from build123d import *

# Parameters (mm, degrees)
SKETCH_W        = 40
SKETCH_H        = 50
PAD_DEPTH       = 7
SKETCH001_R     = 2.5
SKETCH001_R_2   = 5
POCKET_DEPTH    = 7.001
POCKET001_DEPTH = 5
SKETCH003_W     = 11.6
SKETCH003_H     = 1
PAD001_DEPTH    = 50
SKETCH004_R     = 3
POCKET002_DEPTH = 8.001
SKETCH005_R     = 6
POCKET003_DEPTH = 1
CHAMFER_SIZE    = 2.49
FILLET_R        = 4
POCKET004_DEPTH = 8.001
FILLET001_R     = 1


with BuildPart() as part:
    # Sketch → Pad (new body)
    with BuildSketch(Plane.XY):
        with Locations((10, 0)):
            Rectangle(SKETCH_W, SKETCH_H)
    extrude(amount=PAD_DEPTH)

    # Sketch001 (on Face6 of Pad) → Pocket (cut, through all)
    with BuildSketch(Plane.XY.offset(7)):
        with Locations((21.50647, 18.25)):
            Circle(SKETCH001_R)
        with Locations((21.50647, -18.25)):
            Circle(SKETCH001_R)
        with Locations((22, 0)):
            Circle(SKETCH001_R_2)
    extrude(amount=-POCKET_DEPTH, mode=Mode.SUBTRACT)

    # Sketch002 (on Face4 of Pocket) → Pocket001 (cut)
    with BuildSketch(Plane(origin=(0, 0, 0), x_dir=(1, 0, 0), z_dir=(0, 0, -1))):
        Polygon((19.052731, 14), (23.960208, 14), (26.413947, 18.25), (23.960208, 22.5), (19.052731, 22.5), (16.598992, 18.25), align=None)
        Polygon((19.052731, -22.5), (23.960208, -22.5), (26.413947, -18.25), (23.960208, -14), (19.052731, -14), (16.598992, -18.25), align=None)
    extrude(amount=-POCKET001_DEPTH, mode=Mode.SUBTRACT)

    # Sketch003 (on Face1 of Pocket001) → Pad001 (join)
    with BuildSketch(Plane(origin=(0, 25, 0), x_dir=(-1, 0, 0), z_dir=(0, 1, 0))):
        with Locations((0, -0.5)):
            Rectangle(SKETCH003_W, SKETCH003_H)
    extrude(amount=-PAD001_DEPTH)

    # Sketch004 (on Face5 of Pad001) → Pocket002 (cut, through all)
    with BuildSketch(Plane.XY.offset(7)):
        with Locations((0, 15)):
            Circle(SKETCH004_R)
        with Locations((0, -15)):
            Circle(SKETCH004_R)
    extrude(amount=-POCKET002_DEPTH, mode=Mode.SUBTRACT)

    # Sketch005 (on Face5 of Pocket002) → Pocket003 (cut)
    with BuildSketch(Plane.XY.offset(7)):
        with Locations((0, 15)):
            Circle(SKETCH005_R)
        with Locations((0, -15)):
            Circle(SKETCH005_R)
    extrude(amount=-POCKET003_DEPTH, mode=Mode.SUBTRACT)

    # Chamfer
    chamfer_edges = [part.edges().sort_by_distance(p)[0] for p in [
        (-3, -15, 6),
        (-3, 15, 6),
    ]]
    chamfer(chamfer_edges, length=CHAMFER_SIZE)

    # Fillet
    fillet_edges = [part.edges().sort_by_distance(p)[0] for p in [
        (-10, -25, 3.5),
        (30, -25, 3.5),
        (30, 25, 3.5),
        (-10, 25, 3.5),
    ]]
    fillet(fillet_edges, radius=FILLET_R)

    # Sketch006 (on Face1 of Fillet) → Pocket004 (cut, through all)
    with BuildSketch(Plane.XY.offset(7)):
        with BuildLine():
            ThreePointArc((-10, 15), (-6.785937, 6.309375), (0, 0))
            ThreePointArc((0, 0), (-6.785937, -6.309375), (-10, -15))
            Line((-10, 15), (-10, -15))
        make_face()
    extrude(amount=-POCKET004_DEPTH, mode=Mode.SUBTRACT)

    # Fillet001
    fillet001_edges = [part.edges().sort_by_distance(p)[0] for p in [
        (30, 0, 7),
    ]]
    fillet(fillet001_edges, radius=FILLET001_R)


solid = part.part
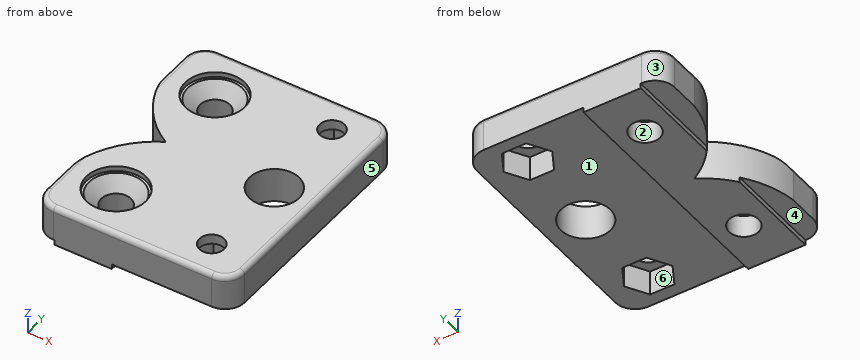
The model under review builds one solid part; all positions refer to its coordinate system, in mm. Face numbers are marked on the shaded views. A direction names the side the tool comes from. Coordinates: 2 decimals unless noted, no trailing zeros. Write each loop counter-clockwise with the first axis right and the second up, starting at its lowest first coordinate (ties: lowest second). Pieces come first, ordered by that corner, then holes. Notation, with made-up numbers: (11, -32.75) - (39, -32.75) arc R8 cw to (39, -23.75) - close; hole circle Ø7 at (85, 59.5). An arc over 180 degrees is marked (long way). Answer as a JSON object with one key per item and string values. Group by question number.
1. Clearance check with flat-ended pins moving along their axes: pin 1 Ø3.5 at (x, y) = (-8, -11) entering from -Z; pin 2 Ø0.5 at (y, z) = (-17, -0.5) entering from -X; pin 3 Ø4.5 at (x, y) = (21.51, 18.25) entering from +Z. State where each tip first meets the part, or that it passes through.
2. To check wall thickness, follow probe 1 along Y at (x, z) = (22, 1.5); probe 2 along Y at (x, z) = (19, 1.5); probe 3 along Z at (x, y) = (15, -17). State the ranges of each line that lie inside material, in increasing order.
3. Add section A-A (z = 1). Give the boundary of the cut face in (x, y), plus the area to 3 significant figures.
4. Add section D-D (x = 20.5). Give the boundary of the cut face in (y, z), plus the area to 3 significant figures.
5. Machinability: for the marked faces 4, 5 and 6, which of the approach directions +Z, -Z, +X, -X, +Y, -Y give a long, thin tool a straight path to every point of the face, cutting with its end or side? Answer none if there is none.
6. Mouldability with a two-part tool opening along X and no side actions: class the marked faces 1, 2 and 3 as pulls with the +X half, pulls with the -X half, needs draft (parallel to the pull), parting line crosses it, or undercut.
7. Add section B-B (x = 15). Give the boundary of the cut face in (y, z).
8. Add section C-C (y = -4). Give the boundary of the cut face in (x, z), plus the area to 3 significant figures.
Findings:
{
 "1": {"pin 1": "z = 0", "pin 2": "x = -5.8", "pin 3": "through"},
 "2": {"probe 1": "-25 to -22.5, -14 to -5, 5 to 14, 22.5 to 25", "probe 2": "-25 to -22.41, -14.09 to -4, 4 to 14.09, 22.41 to 25", "probe 3": "0 to 7"},
 "3": {"outline": "(-10, -21) arc R4 ccw to (-6, -25) - (26, -25) arc R4 ccw to (30, -21) - (30, 21) arc R4 ccw to (26, 25) - (-6, 25) arc R4 ccw to (-10, 21) - (-10, 15) arc R20 ccw to (0, 0) arc R20 ccw to (-10, -15) - close; hole circle Ø6 at (0, -15); hole circle Ø6 at (0, 15); hole (16.6, -18.25) - (19.05, -22.5) - (23.96, -22.5) - (26.41, -18.25) - (23.96, -14) - (19.05, -14) - close; hole (16.6, 18.25) - (19.05, 14) - (23.96, 14) - (26.41, 18.25) - (23.96, 22.5) - (19.05, 22.5) - close; hole circle Ø10 at (22, 0)", "area": "1,630 mm²"},
 "4": {"outline": "(-25, 0) - (-22.5, 0) - (-22.5, 5) - (-20.54, 5) - (-20.54, 7) - (-24, 7) arc R1 ccw to (-25, 6) - close; (-15.96, 5) - (-14, 5) - (-14, 0) - (-4.77, 0) - (-4.77, 7) - (-15.96, 7) - close; (4.77, 0) - (14, 0) - (14, 5) - (15.96, 5) - (15.96, 7) - (4.77, 7) - close; (20.54, 5) - (22.5, 5) - (22.5, 0) - (25, 0) - (25, 6) arc R1 ccw to (24, 7) - (20.54, 7) - close", "area": "179 mm²"},
 "5": {"face 4": "-Z, -X, +Y, -Y", "face 5": "+Z, -Z, +X, +Y, -Y", "face 6": "-Z"},
 "6": {"face 1": "needs draft", "face 2": "undercut", "face 3": "pulls with the -X half"},
 "7": {"outline": "(-25, 0) - (25, 0) - (25, 6) arc R1 ccw to (24, 7) - (-24, 7) arc R1 ccw to (-25, 6) - close"},
 "8": {"outline": "(-4.99, -1) - (5.8, -1) - (5.8, 0) - (19, 0) - (19, 7) - (-4.99, 7) - close; (25, 0) - (30, 0) - (30, 6) arc R1 ccw to (29, 7) - (25, 7) - close", "area": "213 mm²"}
}
